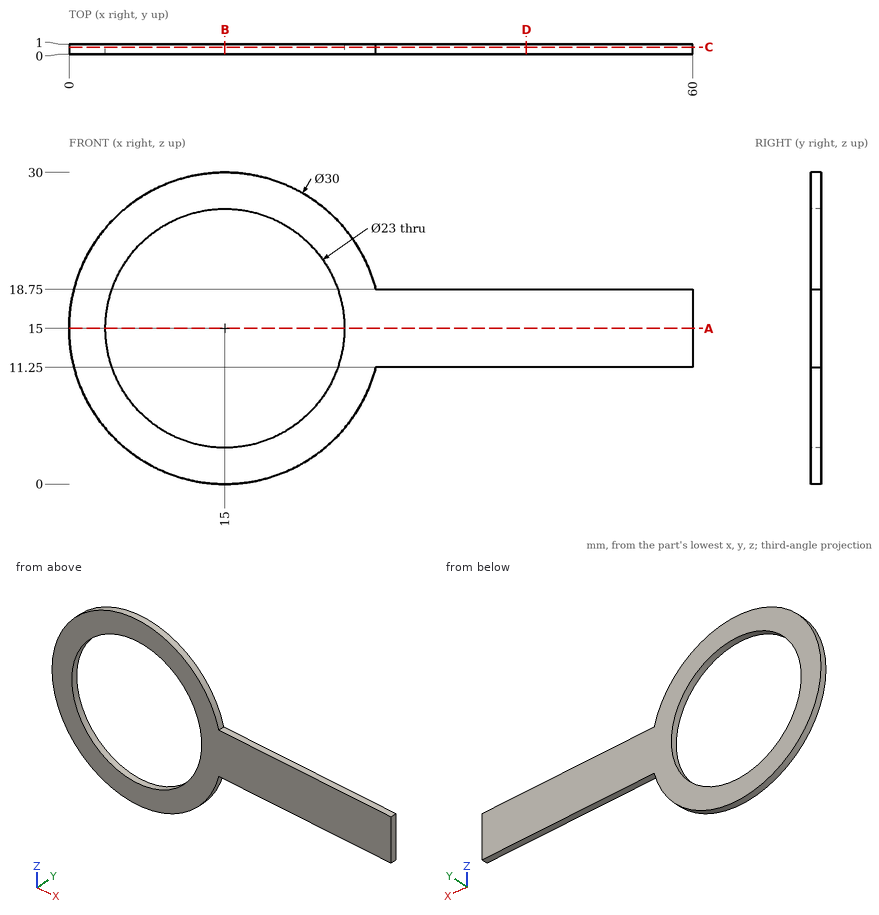
Verification items for this drawing (mm, ordinates from the low corner). Coordinates: 2 decimals unless noted, no trailing zeros. Order: outer loops, then holes, each group sorted by start corner. A loop starts at its lowest first (then second) coordinate and runs counter-clockwise, first axis right, second up. Notation, with made-up numbers: (14.5, -5) - (20.5, -5) arc R34 cw to (20.5, 32) - close; hole circle Ø4 at (48.25, 83). An arc over 180 degrees is marked (long way). Answer in a Markdown table with one row per item. Add a question column.
1. Section check C-C (y = 0.7). Enter the section's corners in (x, z).
2. Section check A-A (z = 15). Enter the section's corners in (x, y).
3. Material ranges on L1, parallel to X at y = 0.6, z = 14.5; L2, parallel to Z at x = 15, y = 0.6; L3, parallel to Z at x = 46, y = 0.5, recorded low to high. Write a range as [from, to].
4. Section check D-D (x = 44). Enter the section's corners in (y, z).
5. Section check B-B (x = 15). Enter the section's corners in (y, z).
6. Gauge pin test, flat ends, axial feed: pin 1 Ø0.5 at (x, y) = (45.5, 0.5) entering from -Z; pin 2 Ø0.5 at (x, y) = (49.5, 0.5) entering from +Z. Record the tip position at first contact, or that the pin passes through.
Data:
| question | item | result |
|---|---|---|
| 1 | outline | (29.52, 11.25) - (60, 11.25) - (60, 18.75) - (29.52, 18.75) arc R15 ccw (long way) to start; hole circle Ø23 at (15, 15) |
| 2 | outline | (0, 0) - (3.5, 0) - (3.5, 1) - (0, 1) - close; (26.5, 0) - (60, 0) - (60, 1) - (26.5, 1) - close |
| 3 | L1 | x = [0.01, 3.51], [26.49, 60] |
| 3 | L2 | z = [0, 3.5], [26.5, 30] |
| 3 | L3 | z = [11.25, 18.75] |
| 4 | outline | (0, 11.25) - (1, 11.25) - (1, 18.75) - (0, 18.75) - close |
| 5 | outline | (0, 0) - (1, 0) - (1, 3.5) - (0, 3.5) - close; (0, 26.5) - (1, 26.5) - (1, 30) - (0, 30) - close |
| 6 | pin 1 | stops at z = 11.25 |
| 6 | pin 2 | stops at z = 18.75 |
